The listing builds one solid part. Answer for the finished solid, in the listing's coordinates (mm). Coordinates: 2 decimals unless noted, no trailing zeros. Loops run counter-clockwise (first coordinate to the right, second up) from the corner with the lowest first, then second, coordinate; pieces in that order, holes last. Notation, with made-up numbers: (-4.75, 26) - (20.25, 26) arc R31 ccw to (20.25, 64) - close; hole circle Ø2 at (44, 10.25). An arc over 180 degrees is marked (long way). Return JSON: item names as keys, results as strings. Group by question number.
1. Section B-B (z = 16.75) is taken. State how many separate pieces and enclosed holes the cut face has, and give its area (3 significant figures).
2. Find the intervals of material crossed by line 1 along Y through (x, z) = (267.5, 14.75); line 2 along X through (y, z) = (42.5, 2.75); line 3 along X through (y, z) = (19.5, 13.5), in increasing order.
3. Section D-D (x = 200) is taken. Write down the section's boundary in (y, z).
4. Each of these flat-tipped pins is pushed along its axis until it touches: P1, Ø3, axis at x = 159, y = 42, coming from the +Z side; P2, Ø13, axis at x = 160, y = 25, coming from the +Z side; P3, Ø3, axis at x = 268, y = 9.5, coming from the -Z side. Where does it stop, or does it pass through?
5. Section A-A (x = 35) is taken. Write down the section's boundary in (y, z), and give its area (3 significant figures).
```python
from build123d import *

# Parameters (mm, degrees)
F0_W     = 320
F0_H     = 50
F1_DEPTH = 20
F2_R     = 3
F2_R_2   = 4
F3_DEPTH = 20
F4_R     = 7.5
F5_DEPTH = 9
F6_R     = 5
F7_DEPTH = 7
F8_R     = 3
F9_DEPTH = 10


with BuildPart() as f1:
    # F0 (on Top) → F1 (new body)
    with BuildSketch(Plane.XY):
        with Locations((160, 25)):
            Rectangle(F0_W, F0_H)
    extrude(amount=F1_DEPTH)

    # F2 (on face) → F3 (cut)
    with BuildSketch(Plane.XY.offset(20)):
        with Locations((17.5, 42.5)):
            Circle(F2_R)
        with Locations((17.5, 7.5)):
            Circle(F2_R)
        with Locations((52.5, 7.5)):
            Circle(F2_R)
        with Locations((52.5, 42.5)):
            Circle(F2_R)
        with Locations((35, 25)):
            Circle(F2_R_2)
        with Locations((95, 25)):
            Circle(F2_R_2)
        with Locations((160, 25)):
            Circle(F2_R_2)
        with Locations((225, 25)):
            Circle(F2_R_2)
        with Locations((285, 25)):
            Circle(F2_R_2)
        with Locations((267.5, 42.5)):
            Circle(F2_R)
        with Locations((302.5, 42.5)):
            Circle(F2_R)
        with Locations((302.5, 7.5)):
            Circle(F2_R)
        with Locations((267.5, 7.5)):
            Circle(F2_R)
    extrude(amount=-F3_DEPTH, mode=Mode.SUBTRACT)

    # F4 (on face) → F5 (cut)
    with BuildSketch(Plane.XY.offset(20)):
        with Locations((35, 25)):
            Circle(F4_R)
        with Locations((95, 25)):
            Circle(F4_R)
        with Locations((160, 25)):
            Circle(F4_R)
        with Locations((225, 25)):
            Circle(F4_R)
        with Locations((285, 25)):
            Circle(F4_R)
    extrude(amount=-F5_DEPTH, mode=Mode.SUBTRACT)

    # F6 (on face) → F7 (cut)
    with BuildSketch(Plane(origin=(0, 0, 0), x_dir=(1, 0, 0), z_dir=(0, 0, -1))):
        with Locations((17.5, -7.5)):
            Circle(F6_R)
        with Locations((17.5, -42.5)):
            Circle(F6_R)
        with Locations((52.5, -42.5)):
            Circle(F6_R)
        with Locations((52.5, -7.5)):
            Circle(F6_R)
        with Locations((267.5, -7.5)):
            Circle(F6_R)
        with Locations((302.5, -7.5)):
            Circle(F6_R)
        with Locations((302.5, -42.5)):
            Circle(F6_R)
        with Locations((267.5, -42.5)):
            Circle(F6_R)
    extrude(amount=-F7_DEPTH, mode=Mode.SUBTRACT)

    # F8 (on face) → F9 (cut)
    with BuildSketch(Plane.XY.offset(20)):
        with Locations((120, 42.5)):
            Circle(F8_R)
        with Locations((120, 7.5)):
            Circle(F8_R)
        with Locations((160, 42.5)):
            Circle(F8_R)
        with Locations((160, 7.5)):
            Circle(F8_R)
        with Locations((200, 42.5)):
            Circle(F8_R)
        with Locations((200, 7.5)):
            Circle(F8_R)
    extrude(amount=-F9_DEPTH, mode=Mode.SUBTRACT)


solid = f1.part
```
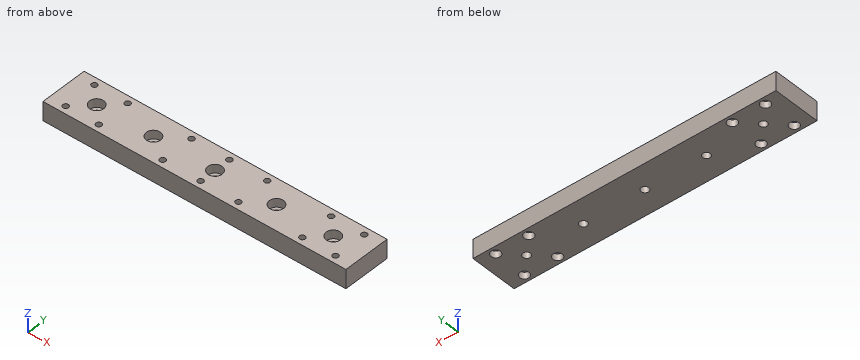
The answers:
{
 "1": {"separate pieces": "1", "enclosed holes": "19", "area": "14,700 mm2"},
 "2": {"line 1": "y = 0 to 4.5, 10.5 to 39.5, 45.5 to 50", "line 2": "x = 0 to 12.5, 22.5 to 47.5, 57.5 to 262.5, 272.5 to 297.5, 307.5 to 320", "line 3": "x = 0 to 29.9, 40.1 to 89.9, 100.1 to 154.9, 165.1 to 219.9, 230.1 to 279.9, 290.1 to 320"},
 "3": {"outline": "(0, 0) - (50, 0) - (50, 20) - (45.5, 20) - (45.5, 10) - (39.5, 10) - (39.5, 20) - (10.5, 20) - (10.5, 10) - (4.5, 10) - (4.5, 20) - (0, 20) - close"},
 "4": {"P1": "stops at z = 10", "P2": "stops at z = 11", "P3": "stops at z = 7"},
 "5": {"outline": "(0, 0) - (21, 0) - (21, 11) - (17.5, 11) - (17.5, 20) - (0, 20) - close; (29, 0) - (50, 0) - (50, 20) - (32.5, 20) - (32.5, 11) - (29, 11) - close", "area": "777 mm2"}
}
